Can you work these out from the drawing? Everything is in mm from the part's minimum corner. A direction names the side the tool comes from. Give positions to 0.01 mm unless a question says otherwise; leave off trailing zeros. Order: outer loops, then holes, each group sorted by start corner. A loop starts at its lowest first (then second) coordinate and runs counter-clockwise, first axis right, second up. Notation, with made-up numbers: (-34.75, -9) - (17.25, -9) arc R14 ccw to (17.25, 9) - close; hole circle Ø3 at (71.25, -38.75). An arc over 180 degrees is marked (long way). Answer as a JSON object with one key per item and string values.
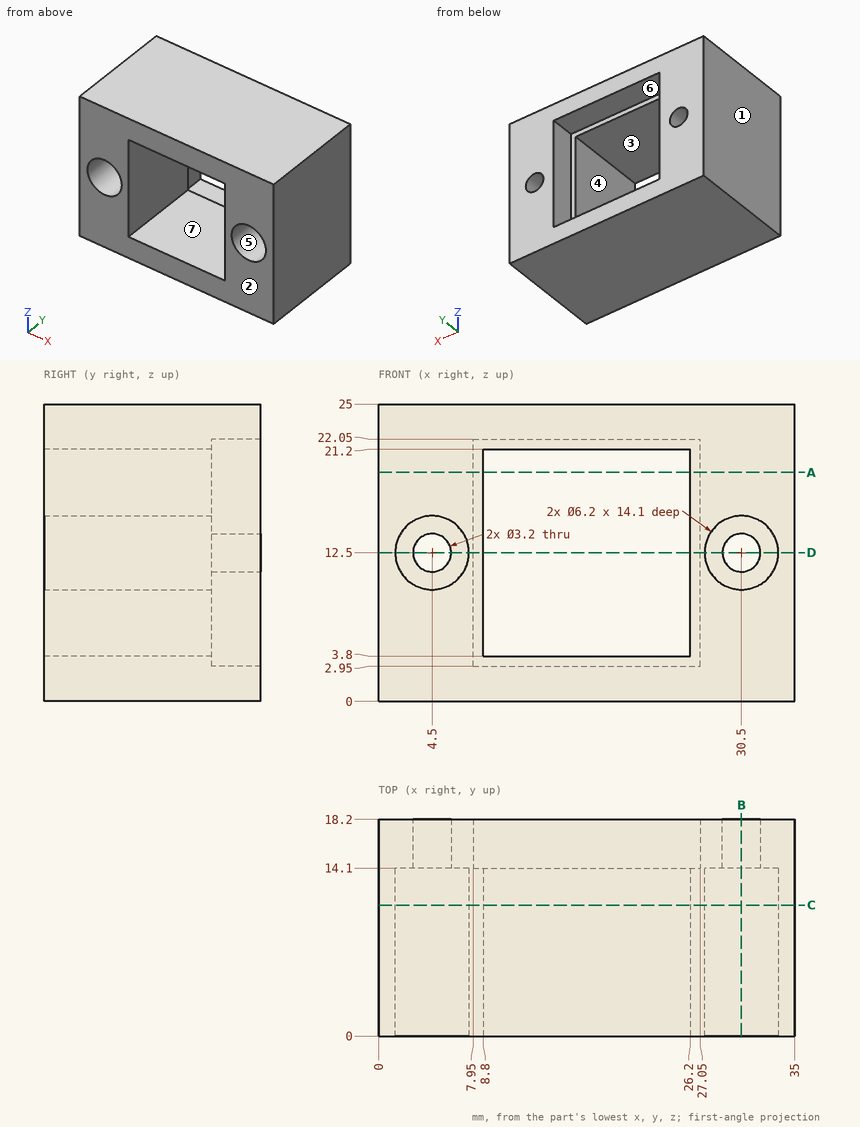
Q1. Which directions (+Z, -Z, +X, -X, +Y, -Y) give clear straight access to the entire face, cutting with the end or side of a thin tool? Please do the marked faces 5, 6 and 7.
Recorded:
{"face 5": "-Y", "face 6": "+Y", "face 7": "+Y, -Y"}
Q2. I'm going to push flat-ended pins straight in: pin 1 Ø10 at (x, y) = (25, 5) entering from -Z; pin 2 Ø1.9 at (x, z) = (5, 12.5) entering from -Y; pin 3 Ø5 at (x, z) = (4.5, 12.5) entering from -Y. Where does each tip first touch, or does it pass through?
Recorded:
{"pin 1": "stops at z = 0", "pin 2": "passes through", "pin 3": "stops at y = 14.1"}
Q3. If we section it at C-C, the plane y = 11: Please give me the cut outline in (x, z).
Recorded:
{"outline": "(0, 0) - (35, 0) - (35, 25) - (0, 25) - close; hole circle Ø6.2 at (4.5, 12.5); hole (8.8, 3.8) - (26.2, 3.8) - (26.2, 21.2) - (8.8, 21.2) - close; hole circle Ø6.2 at (30.5, 12.5)"}
Q4. If we section it at A-A, the plane z = 19.25: Please give me the cut outline in (x, y), then the cut area to 3 significant figures.
Recorded:
{"outline": "(0, 0) - (8.8, 0) - (8.8, 14.1) - (7.95, 14.1) - (7.95, 18.2) - (0, 18.2) - close; (26.2, 0) - (35, 0) - (35, 18.2) - (27.05, 18.2) - (27.05, 14.1) - (26.2, 14.1) - close", "area": "313 mm^2"}
Q5. I need wall thicknesses on L1, parallel to X at y = 11.25, z = 20; L2, parallel to Z at x = 4.5, y = 3; L3, parallel to Z at x = 14.5, y = 11. Which ranges of each line are inside material? Lowest first, please.
Recorded:
{"L1": "x = 0 to 8.8, 26.2 to 35", "L2": "z = 0 to 9.4, 15.6 to 25", "L3": "z = 0 to 3.8, 21.2 to 25"}
Q6. If we section it at B-B, the plane x = 30.5: Please give me the cut outline in (y, z).
Recorded:
{"outline": "(0, 0) - (18.2, 0) - (18.2, 10.9) - (14.1, 10.9) - (14.1, 9.4) - (0, 9.4) - close; (0, 15.6) - (14.1, 15.6) - (14.1, 14.1) - (18.2, 14.1) - (18.2, 25) - (0, 25) - close"}
Q7. We'd pull the mould along X, two halves only. Please class the marked faces 1, 2, 3 and 4: released by +X, released by -X, zero draft, split by the parting line, or undercut.
Recorded:
{"face 1": "released by -X", "face 2": "zero draft", "face 3": "undercut", "face 4": "undercut"}
Q8. If we section it at D-D, the plane z = 12.5: Please give me the cut outline in (x, y), then the cut area to 3 significant figures.
Recorded:
{"outline": "(0, 0) - (1.4, 0) - (1.4, 14.1) - (2.9, 14.1) - (2.9, 18.2) - (0, 18.2) - close; (6.1, 14.1) - (7.6, 14.1) - (7.6, 0) - (8.8, 0) - (8.8, 14.1) - (7.95, 14.1) - (7.95, 18.2) - (6.1, 18.2) - close; (26.2, 0) - (27.4, 0) - (27.4, 14.1) - (28.9, 14.1) - (28.9, 18.2) - (27.05, 18.2) - (27.05, 14.1) - (26.2, 14.1) - close; (32.1, 14.1) - (33.6, 14.1) - (33.6, 0) - (35, 0) - (35, 18.2) - (32.1, 18.2) - close", "area": "112 mm^2"}
